```python
from build123d import *

# Parameters (mm, degrees)
BOSS_EXTRUDE1_DEPTH = 190
SKETCH3_W           = 170
SKETCH3_H           = 20
CUT_EXTRUDE1_DEPTH  = 190
SKETCH4_W           = 4
SKETCH4_H           = 5
BOSS_EXTRUDE2_DEPTH = 19.5
SKETCH5_R           = 2.75
CUT_EXTRUDE3_DEPTH  = 10
SKETCH7_W           = 4
SKETCH7_H           = 19.5
BOSS_EXTRUDE3_DEPTH = 3
BOSS_EXTRUDE4_REACH = 195.391
SKETCH8_R           = 2.75
SKETCH8_R_2         = 2.5
SKETCH9_R           = 2.5
CUT_EXTRUDE4_DEPTH  = 194.390796058
SKETCH10_R          = 2
CUT_EXTRUDE5_DEPTH  = 193.792634714


with BuildPart() as part:
    # Sketch2 → Boss-Extrude1 (new body)
    with BuildSketch(Plane.XY):
        Polygon((0, 0), (0, 10), (10, 10), (10, 30), (20, 30), (20, 0), align=None)
    extrude(amount=BOSS_EXTRUDE1_DEPTH)

    # Sketch3 → Cut-Extrude1 (cut)
    with BuildSketch(Plane(origin=(20, 0, 0), x_dir=(0, 0, -1), z_dir=(1, 0, 0))):
        with Locations((-85, 10)):
            Rectangle(SKETCH3_W, SKETCH3_H)
    extrude(amount=-CUT_EXTRUDE1_DEPTH, mode=Mode.SUBTRACT)

    # Sketch4 → Boss-Extrude2 (add)
    with BuildSketch(Plane(origin=(0, 0, 0), x_dir=(-1, 0, 0), z_dir=(0, 0, -1))):
        with Locations((-15, 27.5)):
            Rectangle(SKETCH4_W, SKETCH4_H)
    extrude(amount=BOSS_EXTRUDE2_DEPTH)

    # Sketch5 → Cut-Extrude3 (cut)
    with BuildSketch(Plane.ZY):
        with Locations((180, 5)):
            Circle(SKETCH5_R)
    extrude(amount=-CUT_EXTRUDE3_DEPTH, mode=Mode.SUBTRACT)

    # Sketch7 → Boss-Extrude3 (add)
    with BuildSketch(Plane.XZ.offset(-25)):
        with Locations((15, -9.75)):
            Rectangle(SKETCH7_W, SKETCH7_H)
    extrude(amount=BOSS_EXTRUDE3_DEPTH)

    # Sketch8 → Boss-Extrude4 (add, up to next)
    with BuildSketch(Plane.ZY, mode=Mode.PRIVATE) as boss_extrude4_sk1:
        with Locations((180, 5)):
            Circle(SKETCH8_R)
        with Locations((180, 5)):
            Circle(SKETCH8_R_2, mode=Mode.SUBTRACT)
    boss_extrude4_tool1 = extrude(boss_extrude4_sk1.sketch, amount=-BOSS_EXTRUDE4_REACH, mode=Mode.PRIVATE) - part.part
    add(boss_extrude4_tool1.solids().sort_by_distance((0, 5, 177.327782))[0])

    # Sketch9 → Cut-Extrude4 (cut, through all)
    with BuildSketch(Plane.ZY):
        with Locations((180, 5)):
            Circle(SKETCH9_R)
    extrude(amount=-CUT_EXTRUDE4_DEPTH, mode=Mode.SUBTRACT)

    # Sketch10 → Cut-Extrude5 (cut, through all)
    with BuildSketch(Plane.ZY.offset(-13)):
        with Locations((-9.5, 25)):
            Circle(SKETCH10_R)
    extrude(amount=-CUT_EXTRUDE5_DEPTH, mode=Mode.SUBTRACT)


solid = part.part
```
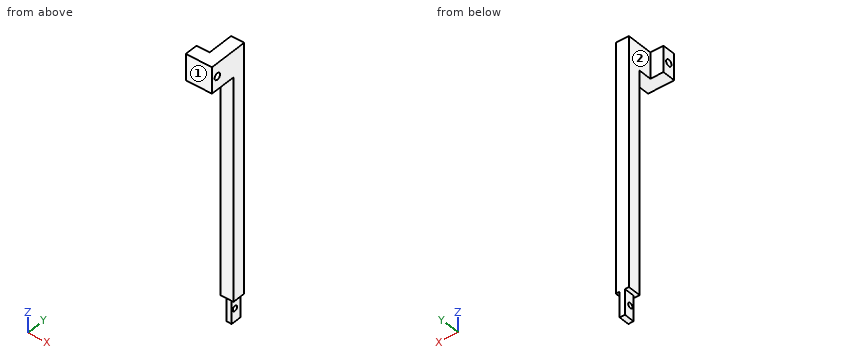
The listing builds one solid part. Answer for the finished solid, in the listing's coordinates (mm). Face numbers are marked on the shaded views. A direction names the side the tool comes from. Coordinates: 2 decimals unless noted, no trailing zeros. Loops run counter-clockwise (first coordinate to the right, second up) from the corner with the lowest first, then second, coordinate; pieces in that order, holes last. Notation, with made-up numbers: (74.25, 45) -> (132.25, 45) arc R8 cw to (132.25, 56) -> close; hole circle Ø11 at (80.25, -4). An arc over 180 degrees is marked (long way). Return JSON: item names as keys, results as strings. Group by question number.
(1) A cutting plane is placed at C-C on y = 25. Write down the section's boundary in (x, z).
(2) Which of the six approach directions +Z, -Z, +X, -X, +Y, -Y give full straight-line access (tool end or side, diameter ignored) to the marked faces 1 and 2?
(3) A cutting plane is placed at D-D on z = -9.5. Write down the section's boundary in (x, y), and give its area (3 significant figures).
(4) A cutting plane is placed at B-B on z = 180. Write down the section's boundary in (x, y), and give its area (3 significant figures).
(5) A cutting plane is placed at A-A on y = 5. Write down the section's boundary in (x, z).
(6) Given pin 1 Ø9 at (y, z) = (24.5, -9) entering from -X; pin 2 Ø8 at (x, z) = (6.5, 34.5) entering from -Y; pin 3 Ø2.5 at (y, z) = (25, -9.5) entering from -X; pin 4 Ø2.5 at (y, z) = (25, -6.5) entering from +X, each flat-ended and moving along its own axis, determine where each tip first touches the part or whether it passes through.
(7) Find the intervals of material crossed by probe 1 along Y at (x, z) = (11.75, 180); probe 2 along Y at (x, z) = (15.25, -9.5); probe 3 along Z at (x, y) = (6, 1.5), in increasing order. Write a range as from..to.
The answers:
{
 "1": {"outline": "(10, 0) -> (13, 0) -> (13, -7.5) -> (17, -7.5) -> (17, 0) -> (20, 0) -> (20, 190) -> (10, 190) -> close; (13, -19.5) -> (17, -19.5) -> (17, -11.5) -> (13, -11.5) -> close"},
 "2": {"face 1": "+Z, -Z, +X, -X, -Y", "face 2": "+Z, -Z, -X, +Y"},
 "3": {"outline": "(13, 22) -> (17, 22) -> (17, 23) -> (13, 23) -> close; (13, 27) -> (17, 27) -> (17, 30) -> (13, 30) -> close", "area": "16.0 mm^2"},
 "4": {"outline": "(0, 0) -> (20, 0) -> (20, 2.5) -> (0, 2.5) -> close; (0, 7.5) -> (20, 7.5) -> (20, 30) -> (10, 30) -> (10, 10) -> (0, 10) -> close", "area": "300 mm^2"},
 "5": {"outline": "(0, 170) -> (20, 170) -> (20, 177.5) -> (0, 177.5) -> close; (0, 182.5) -> (20, 182.5) -> (20, 190) -> (0, 190) -> close"},
 "6": {"pin 1": "stops at x = 13", "pin 2": "stops at y = 20", "pin 3": "passes through", "pin 4": "stops at x = 17"},
 "7": {"probe 1": "y = 0..2.5, 7.5..30", "probe 2": "y = 22..23, 27..30", "probe 3": "z = 170..190"}
}
